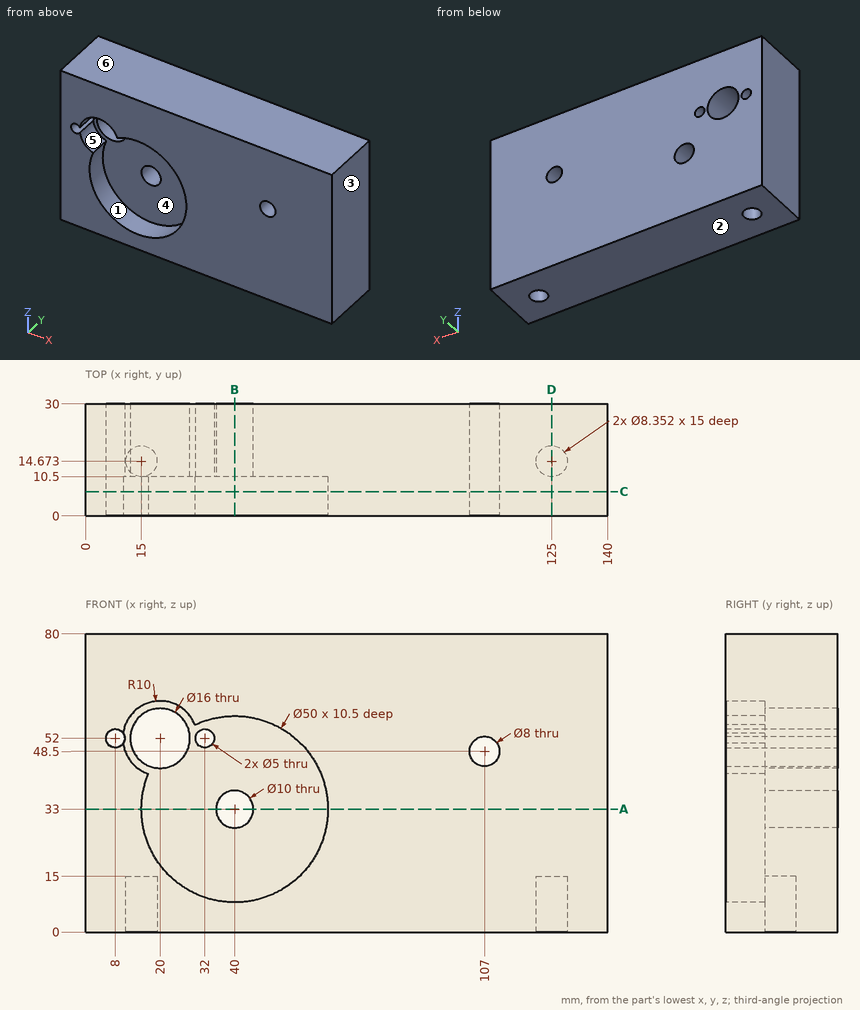
Print and shaded views of the part. All mm, measured from the part's lowest x, y and z. A direction names the side the tool comes from. Round coordinates to 2 decimals unless told otherwise and drop trailing zeros. Write each loop counter-clockwise with the first axis right and the second up, starting at its lowest first coordinate (ties: lowest second). Pieces come first, ordered by that corner, then holes. Notation, with made-up numbers: (16, 43.25) - (57, 43.25) arc R21 cw to (57, 79.25) - close; hole circle Ø1 at (47, 77.25). An arc over 180 degrees is marked (long way). Write each question's results on one line, items separated by ' | '. Start each with the question number.
Item 1: Saw through at B-B (x = 40). Write the cut outline in (y, z).
Item 2: Which spindle directions (+Z, -Z, +X, -X, +Y, -Y) get a long thin tool onto all of the face, cutting with end or side? Do the marked faces 5 and 6. Say none if no direction does.
Item 3: Saw through at A-A (z = 33). Write the cut outline in (x, y), and give its area (3 significant figures).
Item 4: Mould opens along X. For the marked faces 1, 2, 3 and 4 say: pulls with the +X half, pulls with the -X half, needs draft (parallel to the pull), parting line crosses it, or undercut.
Item 5: Saw through at D-D (x = 125). Write the cut outline in (y, z).
Item 6: Drop flat-ended pins along their axis: P1, Ø3, axis at x = 111, y = 22.5, coming from the -Z side; P2, Ø6.5, axis at x = 125, y = 14.67, coming from the -Z side; P3, Ø6, axis at x = 40, z = 33, coming from the +Y side; P4, Ø8, axis at x = 32, z = 52, coming from the -Y side. Give the stop position or say it passes through.
Item 7: Wall check: L1, parallel to Y at x = 125, z = 7.5; L2, parallel to Z at x = 107, y = 21.75; L3, parallel to Z at x = 40, y = 17.5. Give the ranges that are in metal, low to high. Write a range as [from, to].
Item 8: Saw through at C-C (y = 6.5). Write the cut outline in (x, z), and give its area (3 significant figures).
Results are:
1) outline: (0, 0) - (30, 0) - (30, 28) - (10.5, 28) - (10.5, 8) - (0, 8) - close; (0, 58) - (10.5, 58) - (10.5, 38) - (30, 38) - (30, 80) - (0, 80) - close
2) face 5: -Y | face 6: +Z, +X, -X, +Y, -Y
3) outline: (0, 0) - (15, 0) - (15, 10.5) - (35, 10.5) - (35, 30) - (0, 30) - close; (45, 10.5) - (65, 10.5) - (65, 0) - (140, 0) - (140, 30) - (45, 30) - close | area: 3,480 mm²
4) face 1: undercut | face 2: needs draft | face 3: pulls with the +X half | face 4: undercut
5) outline: (0, 0) - (10.5, 0) - (10.5, 15) - (18.85, 15) - (18.85, 0) - (30, 0) - (30, 80) - (0, 80) - close
6) P1: stops at z = 0 | P2: stops at z = 15 | P3: passes through | P4: stops at y = 10.5
7) L1: y = [0, 10.5], [18.85, 30] | L2: z = [0, 44.5], [52.5, 80] | L3: z = [0, 28], [38, 80]
8) outline: (0, 0) - (140, 0) - (140, 80) - (0, 80) - close; hole (10.09, 50.63) arc R10 ccw to (16.88, 42.5) arc R25 ccw (long way) to (29.33, 55.61) arc R10 ccw to (10.09, 53.37) arc R2.5 ccw (long way) to start; hole circle Ø8 at (107, 48.5) | area: 8,950 mm²
